```python
from build123d import *

# Parameters (mm, degrees)
RECPAT_COUNT = 2
RECPAT_ANGLE = 90


with BuildPart() as part:
    # Fillet1: read off the stored shape, not the designer's step
    # Fillet1 outline → Fillet1 (revolve)
    with BuildSketch(Plane.YX):
        with BuildLine():
            Line((4, 6.3), (4, 50.9))
            Line((4, 50.9), (0, 50.9))
            Line((0, 50.9), (0, 3.9))
            Line((0, 3.9), (9.5, 3.9))
            Line((9.5, 3.9), (9.5, 5.9))
            Line((9.5, 5.9), (4.4, 5.9))
            ThreePointArc((4.4, 5.9), (4.117157288, 6.017157288), (4, 6.3))
        make_face()
    revolve(axis=Axis((0, 0, 0), (1, 0, 0)))

    # PanSke → Pan (revolve)
    with BuildSketch(Plane.XY, mode=Mode.PRIVATE) as pan_sk:
        with BuildLine():
            Line((3.9, 8.401785525), (3.9, 0))
            Line((3.9, 0), (0, 0))
            ThreePointArc((0, 0), (1.02252537, 4.631414471), (3.9, 8.401785525))
        make_face()
    revolve(pan_sk.sketch.rotate(Axis((0, 0, 0), (1, 0, 0)), 90), axis=Axis((0, 0, 0), (1, 0, 0)))

    # Sketch3 → Recess section 0
    with BuildSketch(Plane(origin=(0, 0, 0), x_dir=(0, 0, -1), z_dir=(1, 0, 0))):
        with BuildLine():
            Line((-1.08, 4.4), (1.08, 4.4))
            Line((1.08, 4.4), (1.08, -4.4))
            Line((1.08, -4.4), (-1.08, -4.4))
            Line((-1.08, -4.4), (-1.08, 4.4))
        make_face()
    # Sketch4 → Recess section 1
    with BuildSketch(Plane(origin=(4.52, 0, 0), x_dir=(0, 0, -1), z_dir=(1, 0, 0))):
        with BuildLine():
            Line((-1.08, 2.106524682), (1.08, 2.106524682))
            Line((1.08, 2.106524682), (1.08, -2.106524682))
            Line((1.08, -2.106524682), (-1.08, -2.106524682))
            Line((-1.08, -2.106524682), (-1.08, 2.106524682))
        make_face()
    recess = loft(mode=Mode.SUBTRACT)

    # RecPat: Recess ×2 about axis
    recpat_axis = Axis((0, 0, 0), (1, 0, 0))
    for i in range(1, RECPAT_COUNT):
        add(recess.rotate(recpat_axis, i * RECPAT_ANGLE / (RECPAT_COUNT - 1)), mode=Mode.SUBTRACT)

    # RecCorSke → RecessCore (revolve, cut)
    with BuildSketch(Plane.XY, mode=Mode.PRIVATE) as recesscore_sk:
        Polygon((0, 0), (0, 2.252163335), (4.6, 1.9305), (5.227257474, 0), align=None)
    revolve(recesscore_sk.sketch.rotate(Axis((-3.175, 0, 0), (1, 0, 0)), 90), axis=Axis((-3.175, 0, 0), (1, 0, 0)), mode=Mode.SUBTRACT)


solid = part.part
```
Here's how the part is built. I have some questions about the finished solid (model axes, mm). A direction names the side the tool comes from. Round coordinates to 2 decimals unless told otherwise and drop trailing zeros. Write each loop counter-clockwise with the first axis right and the second up, starting at its lowest first coordinate (ties: lowest second). Pieces come first, ordered by that corner, then holes.
Q1. Which directions (+Z, -Z, +X, -X, +Y, -Y) give clear straight access to the entire face, cutting with the end or side of a thin tool? Please do faces 1 (the flat face through (5.9, 2, -4.1)), 2 (the flat face through (2.666, -3.047, -0.015)), 3 (the cylindrical face through (4.91, 4.38, -8.43)).
Q2. If we section it at B-B on x = 29.5: Write out the boundary of the cut face in (y, z).
Q3. If we section it at C-C on y = 6.25: Write out the boundary of the cut face in (x, z).
Q4. If we section it at A-A on z = -6: Write out the boundary of the cut face in (x, y), plus the area to 3 significant figures.
Q5. If we mould it in two halves opening along Y, with no side actions, what happens to faces 4 (the cylindrical face through (28.912, -0.867, -3.905)), 5 (the flat face through (3.9, 4, -8)), 6 (the conical face through (2.59, -1.49, 1.44))? For each: +Y half, -Y half, draft (parallel to the pull), parting line (faces both ways), or undercut.
Q6. Will these pins go through, and if not, where does the flat tip stop? P1, Ø1, axis at y = 7, z = -6.5, coming from the +X side; P2, Ø8, axis at x = 8.5, y = 1, coming from the -Z side; P3, Ø10, axis at x = 39, z = 4, coming from the -Y side; P4, Ø6, axis at x = 38, y = 3, coming from the -Z side.
Q7. Please list where these lines run through material, in increasing order: probe 1 along X at (y, z) = (4.5, -3.5); probe 2 along Y at (x, z) = (15, 3.5); probe 3 along X at (y, z) = (-3.25, 1.5).
Answer below:
1. face 1: +X
1. face 2: -X
1. face 3: +X, -X
2. outline: circle Ø8 at (0, 0)
3. outline: (3.9, -7.15) - (5.9, -7.15) - (5.9, 7.15) - (3.9, 7.15) - (3.9, 5.61) arc R9.05 ccw to (3.9, -5.61) - close
4. outline: (3.9, -7.37) - (5.9, -7.37) - (5.9, 7.37) - (3.9, 7.37) - (3.9, 5.88) arc R9.22 ccw to (3.9, -5.88) - close
4. area: 46.5 mm2
5. face 4: parting line
5. face 5: draft
5. face 6: undercut
6. P1: stops at x = 5.9
6. P2: stops at z = -9.5
6. P3: stops at y = -4
6. P4: stops at z = -4
7. probe 1: x = 1.59 to 5.9
7. probe 2: y = -1.94 to 1.94
7. probe 3: x = 0.6 to 50.9
